Check sheet for the modelled part. Datum: model origin and axes. Units: mm. A direction names the side the tool comes from. Coordinates: 2 decimals unless noted, no trailing zeros. Loops run counter-clockwise (first coordinate to the right, second up) from the corner with the lowest first, then second, coordinate; pieces in that order, holes last.
```python
from build123d import *

# Parameters (mm, degrees)
SKETCH1_W           = 80
SKETCH1_H           = 160
BOSS_EXTRUDE1_DEPTH = 2
SKETCH2_W           = 80
SKETCH2_H           = 160
SKETCH2_W_2         = 76
SKETCH2_H_2         = 156
BOSS_EXTRUDE2_DEPTH = 130
SKETCH3_W           = 62
SKETCH3_H           = 18
CUT_EXTRUDE1_DEPTH  = 2
SKETCH5_W           = 76
SKETCH5_H           = 29
CUT_EXTRUDE2_DEPTH  = 2
SKETCH7_W           = 76
SKETCH7_H           = 10
BOSS_EXTRUDE3_DEPTH = 20
CHAMFER1_SIZE       = 17
FILLET1_R           = 10


with BuildPart() as part:
    # Sketch1 → Boss-Extrude1 (new body)
    with BuildSketch(Plane.XY):
        Rectangle(SKETCH1_W, SKETCH1_H)
    extrude(amount=BOSS_EXTRUDE1_DEPTH)

    # Sketch2 → Boss-Extrude2 (add)
    with BuildSketch(Plane.XY.offset(2)):
        Rectangle(SKETCH2_W, SKETCH2_H)
        Rectangle(SKETCH2_W_2, SKETCH2_H_2, mode=Mode.SUBTRACT)
    extrude(amount=BOSS_EXTRUDE2_DEPTH)

    # Sketch3 → Cut-Extrude1 (cut)
    with BuildSketch(Plane.XZ.offset(80)):
        with Locations((0, 11)):
            Rectangle(SKETCH3_W, SKETCH3_H)
    extrude(amount=-CUT_EXTRUDE1_DEPTH, mode=Mode.SUBTRACT)

    # Sketch5 → Cut-Extrude2 (cut)
    with BuildSketch(Plane(origin=(0, 80, 0), x_dir=(1, 0, 0), z_dir=(0, 1, 0))):
        with Locations((0, -16.5)):
            Rectangle(SKETCH5_W, SKETCH5_H)
    extrude(amount=-CUT_EXTRUDE2_DEPTH, mode=Mode.SUBTRACT)

    # Sketch7 → Boss-Extrude3 (add)
    with BuildSketch(Plane(origin=(0, -78, 0), x_dir=(1, 0, 0), z_dir=(0, 1, 0))):
        with Locations((0, -25)):
            Rectangle(SKETCH7_W, SKETCH7_H)
    extrude(amount=BOSS_EXTRUDE3_DEPTH)

    # Chamfer1
    # the kernel refuses this chamfer: 17 mm, written as the material it takes off along each edge
    with BuildSketch(Plane(origin=(38, -58, 30), x_dir=(0, 0.027495876610586237, -0.9996219169112966), z_dir=(-1, 0, 0))) as chamfer1_piece_1:
        Polygon((CHAMFER1_SIZE * 0.999621916911, CHAMFER1_SIZE * 0.0274958766106), (-CHAMFER1_SIZE * 0.0274958766106, CHAMFER1_SIZE * 0.999621916911), (0, 0), align=None)
    extrude(amount=76, mode=Mode.SUBTRACT)

    # Fillet1
    # the kernel refuses this fillet: 10 mm, written as the material it takes off along each edge
    with BuildSketch(Plane(origin=(38, -75, 30), x_dir=(0, -1.0, 2.265447089177998e-12), z_dir=(-1, 0, 0))) as fillet1_piece_1:
        with BuildLine():
            CenterArc((4.216391769, -9.925743854), FILLET1_R, 96.986713585, 38.013286415)
            Line((-2.854676043, -2.854676043), (0, 0))
            Line((0, 0), (3, 0))
        make_face()
    extrude(amount=76, mode=Mode.SUBTRACT)


solid = part.part
```
1) Section check D-D on z = 43.5. Enter the section's corners in (x, y).
Answer sheet:
outline: (-40, -80) - (40, -80) - (40, 80) - (-40, 80) - close; hole (-38, -78) - (38, -78) - (38, 78) - (-38, 78) - close
2) Depth check by flat-ended pin: pin 1 (5.5 mm diameter, centred on x = -34, z = 6.5, fed in from +Y); pin 2 (2 mm diameter, centred on x = 5.5, y = -34.5, fed in from -Z); pin 3 (23 mm diameter, centred on x = 5, y = -13.5, fed in from +Z). Enter the tip coordinate at first touch or a pass-through.
Answer sheet:
pin 1: stops at y = -78
pin 2: stops at z = 0
pin 3: stops at z = 2
3) Set-up check for faces 1 (the flat face through (-1, -78, 80)), 2 (the flat face through (1, -69, 24)), 3 (the flat face through (34, -78, 11)), 4 (the flat face through (40, -1, 65)): record each of +Z, -Z, +X, -X, +Y, -Y from which the full face is reachable in a straight line by a thin tool's end or side.
Answer sheet:
face 1: +Z
face 2: +Z, +Y
face 3: +Y
face 4: +Z, -Z, +X, +Y, -Y
4) Section check C-C on y = -32.5. Enter the section's corners in (x, z).
Answer sheet:
outline: (-40, 0) - (40, 0) - (40, 132) - (38, 132) - (38, 2) - (-38, 2) - (-38, 132) - (-40, 132) - close
5) Mould release check, pull along Z, two halves, no side actions. Record for faces 5 (the flat face through (-35, -78, 11)), 6 (the cylindrical face through (0.532, -74.876, 29.083)), 7 (the flat face through (-1, -80, 65)): +Z half, -Z half, draft (parallel to the pull), parting line (faces both ways), or undercut.
Answer sheet:
face 5: undercut
face 6: +Z half
face 7: draft
6) Section check A-A on x = 5.5. Enter the section's corners in (y, z), plus the area to 3 significant figures.
Answer sheet:
outline: (-80, 0) - (80, 0) - (80, 2) - (-80, 2) - close; (-80, 20) - (-65, 20) - (-72.15, 27.15) arc R10 ccw to (-78, 30) - (-78, 132) - (-80, 132) - close; (78, 31) - (80, 31) - (80, 132) - (78, 132) - close
area: 824 mm2
7) Scan lines: line 1 (X direction, y = -70, z = 51.5); line 2 (Y direction, x = -12, z = 52.5); line 3 (Z direction, x = 3, y = 64). Record each from-to range of solid material in increasing order.
Answer sheet:
line 1: x = -40 to -38, 38 to 40
line 2: y = -80 to -78, 78 to 80
line 3: z = 0 to 2
8) Section check B-B on z = 16. Enter the section's corners in (x, y), plus the area to 3 significant figures.
Answer sheet:
outline: (-40, -80) - (-31, -80) - (-31, -78) - (-38, -78) - (-38, 80) - (-40, 80) - close; (31, -80) - (40, -80) - (40, 80) - (38, 80) - (38, -78) - (31, -78) - close
area: 668 mm2
